Input: part model. Units: mm. Frame: model coordinates. A direction names the side the tool comes from. Give positions to 0.01 mm unless a question says otherwise; leave off trailing zeros. Answer as CSV lines item,"result". Start each with the question number.
from build123d import *

# Parameters (mm, degrees)
SKETCH1_W                                        = 300
SKETCH1_H                                        = 200
BOSS_EXTRUDE1_DEPTH                              = 20
FILLET1_R                                        = 10
CBORE_FOR_M3_PAN_HEAD_MACHINE_SCREW1_D           = 3.4
CBORE_FOR_M3_PAN_HEAD_MACHINE_SCREW1_CBORE_D     = 7
CBORE_FOR_M3_PAN_HEAD_MACHINE_SCREW1_CBORE_DEPTH = 2.4
F_5_0_5_DIAMETER_HOLE1_D                         = 5
F_2_0_2_DIAMETER_HOLE1_D                         = 2
F_2_0_2_DIAMETER_HOLE1_DEPTH                     = 10
F_2_0_2_DIAMETER_HOLE1_TIP                       = 0.600860619


with BuildPart() as part:
    # Sketch1 → Boss-Extrude1 (new body)
    with BuildSketch(Plane(origin=(0, 0, 0), x_dir=(1, 0, 0), z_dir=(0, 1, 0))):
        Rectangle(SKETCH1_W, SKETCH1_H)
    extrude(amount=BOSS_EXTRUDE1_DEPTH)

    # Fillet1
    fillet1_edges = [part.edges().sort_by_distance(p)[0] for p in [
        (-150, 10, -100),
        (150, 10, -100),
        (150, 10, 100),
        (-150, 10, 100),
    ]]
    fillet(fillet1_edges, radius=FILLET1_R)

    # CBORE for M3 Pan Head Machine Screw1 (through all)
    with Locations(Plane(origin=(0, 20, 0), x_dir=(1, 0, 0), z_dir=(0, 1, 0))):
        with Locations((-30, 0), (0, -30), (30, 0), (0, 30)):
            CounterBoreHole(CBORE_FOR_M3_PAN_HEAD_MACHINE_SCREW1_D / 2, CBORE_FOR_M3_PAN_HEAD_MACHINE_SCREW1_CBORE_D / 2, CBORE_FOR_M3_PAN_HEAD_MACHINE_SCREW1_CBORE_DEPTH)

    # Ø5.0 (5) Diameter Hole1 (through all)
    with Locations(Plane(origin=(0, 20, 0), x_dir=(1, 0, 0), z_dir=(0, 1, 0))):
        with Locations((-140, 90), (140, 90), (140, -90), (-140, -90)):
            Hole(F_5_0_5_DIAMETER_HOLE1_D / 2)

    # Ø2.0 (2) Diameter Hole1
    with Locations(Plane(origin=(0, 0, 0), x_dir=(-1, 0, 0), z_dir=(0, -1, 0))):
        with Locations((129.008456627, -60.281417871), (123.889747092, -7.883242209), (95.98974887, -7.893204139), (80.707888413, -58.698663894)):
            Hole(F_2_0_2_DIAMETER_HOLE1_D / 2, depth=F_2_0_2_DIAMETER_HOLE1_DEPTH)
            with Locations((0, 0, -(F_2_0_2_DIAMETER_HOLE1_DEPTH + F_2_0_2_DIAMETER_HOLE1_TIP / 2))):  # 118° drill point
                Cone(0, F_2_0_2_DIAMETER_HOLE1_D / 2, F_2_0_2_DIAMETER_HOLE1_TIP, mode=Mode.SUBTRACT)


solid = part.part
1) Contact query for flat-ended pins moving along their axis: P1, Ø1.8, axis at x = -123.89, z = 7.88, coming from the -Y side; P2, Ø5.5, axis at x = 30, z = 0, coming from the +Y side. Output: stop coordinate, or through.
2) Pull-direction query (Z, two-part tool) for faces 3 (the flat face through (150, 10, 1)), 4 (the cylindrical face through (146.99, 10.14, 97.15)), 5 (the flat face through (29, 17.6, 2)); classes: +Z half, -Z half, draft (parallel to the pull), parting line (faces both ways), or undercut.
3) Material intervals for line 1 (Z direction, x = -140, y = 15.75); line 2 (Z direction, x = 30, y = 4.5); line 3 (X direction, y = 5.25, z = 30), sorted ascending. Write a range as from..to.
4) Reachability of faces 1 (the flat face through (-2, 10, -100)), 2 (the cylindrical face through (-26.66, 18.82, -1.05)) from +Z, -Z, +X, -X, +Y, -Y: full face, straight path, thin tool, end or side. Return the list, or none.
Numbers:
1,P1,"stops at y = 10.06"
1,P2,"stops at y = 17.6"
2,face 3,"draft"
2,face 4,"+Z half"
2,face 5,"undercut"
3,line 1,"z = -100..-92.5, -87.5..87.5, 92.5..100"
3,line 2,"z = -100..-1.7, 1.7..100"
3,line 3,"x = -150..-1.7, 1.7..150"
4,face 1,"-Z, +X, -X, +Y, -Y"
4,face 2,"+Y"
